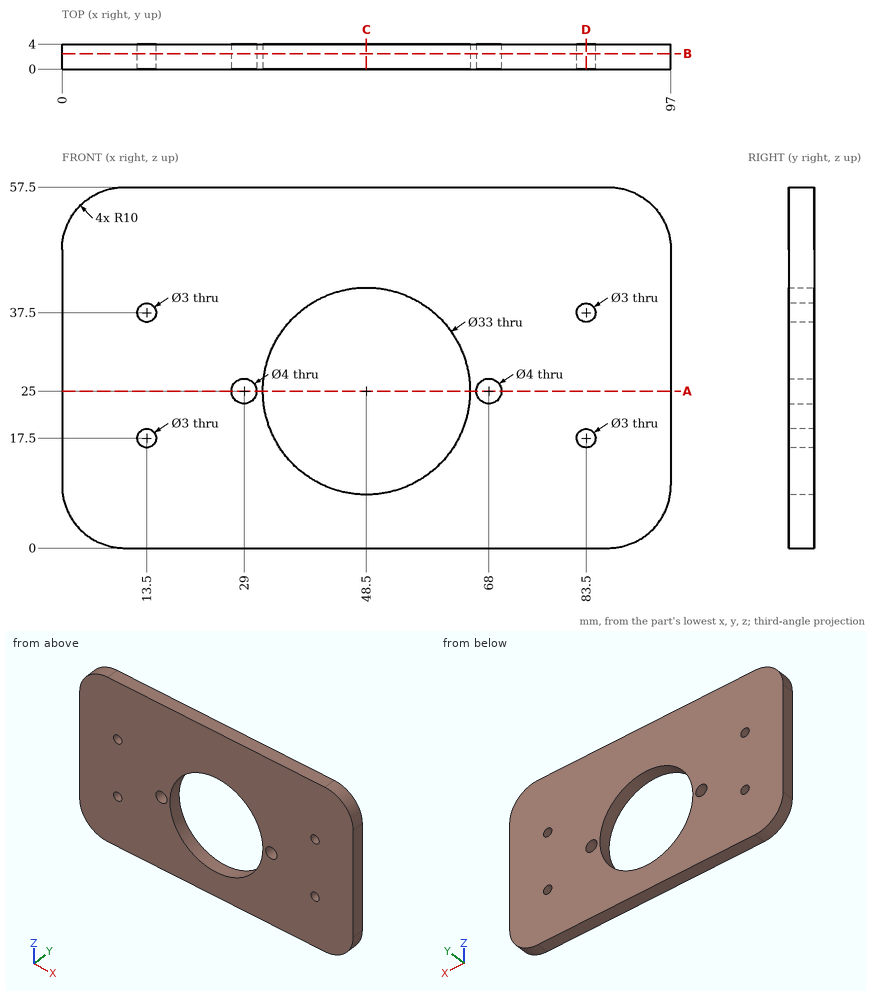
Answer from the drawing. Dimensions are ordinates in mm from the lowest x, y and z of the part. Give positions to 0.01 mm unless a question says otherwise; leave off trailing zeros. Loops run counter-clockwise (first coordinate to the right, second up) from the corner with the lowest first, then second, coordinate; pieces in that order, holes last. Notation, with made-up numbers: M 15.5,32 L 54.5,32 A15 cw 54.5,40 Z; hole C -37,19.25 d1. An arc over 180 degrees is marked long. One line per item, written item: value.
Q1. A cutting plane is placed at D-D on x = 83.5. Determine the outline of the cut face in (y, z).
Working result:
outline: M 0,0 L 4,0 L 4,16 L 0,16 Z; M 0,19 L 4,19 L 4,36 L 0,36 Z; M 0,39 L 4,39 L 4,57.5 L 0,57.5 Z
Q2. A cutting plane is placed at B-B on y = 2.45. Determine the outline of the cut face in (x, z), then the cut area to 3 significant figures.
Working result:
outline: M 0,10 A10 ccw 10,0 L 87,0 A10 ccw 97,10 L 97,47.5 A10 ccw 87,57.5 L 10,57.5 A10 ccw 0,47.5 Z; hole C 13.5,17.5 d3; hole C 13.5,37.5 d3; hole C 29,25 d4; hole C 48.5,25 d33; hole C 68,25 d4; hole C 83.5,17.5 d3; hole C 83.5,37.5 d3
area: 4,580 mm^2
Q3. A cutting plane is placed at A-A on z = 25. Determine the outline of the cut face in (x, y), then the cut area to 3 significant figures.
Working result:
outline: M 0,0 L 27,0 L 27,4 L 0,4 Z; M 31,0 L 32,0 L 32,4 L 31,4 Z; M 65,0 L 66,0 L 66,4 L 65,4 Z; M 70,0 L 97,0 L 97,4 L 70,4 Z
area: 224 mm^2
Q4. A cutting plane is placed at C-C on x = 48.5. Determine the outline of the cut face in (y, z), then the cut area to 3 significant figures.
Working result:
outline: M 0,0 L 4,0 L 4,8.5 L 0,8.5 Z; M 0,41.5 L 4,41.5 L 4,57.5 L 0,57.5 Z
area: 98.0 mm^2
Q5. Find the intervals of material crossed by line 1 (Z direction, x = 83.5, y = 2.55); line 2 (X direction, y = 3.2, z = 17.5); line 3 (X direction, y = 1.15, z = 37.5), in increasing order. Write a range as from..to.
Working result:
line 1: z = 0..16, 19..36, 39..57.5
line 2: x = 0..12, 15..33.8, 63.2..82, 85..97
line 3: x = 0..12, 15..37.73, 59.27..82, 85..97
